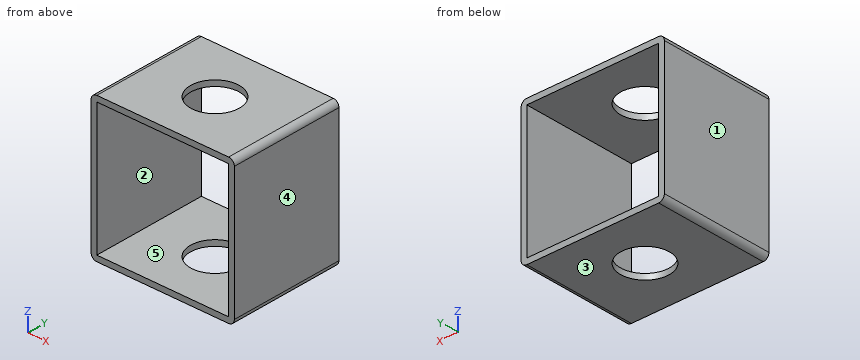
```python
from build123d import *

# Parameters (mm, degrees)
SKETCH1_W               = 46
SKETCH1_H               = 46
EXTRUDE_THIN1_DEPTH     = 20
CUT_EXTRUDE1_DEPTH      = 58.697486947
CUT_EXTRUDE1_DEPTH_BACK = 58.697486947
SKETCH2_R               = 8.5


with BuildPart() as part:
    # Sketch1 → Extrude-Thin1 (new, symmetric)
    with BuildSketch(Plane(origin=(0, 0, 0), x_dir=(1, 0, 0), z_dir=(0, 1, 0))):
        with BuildLine():
            Line((-23, 25), (23, 25))
            ThreePointArc((23, 25), (24.414213562, 24.414213562), (25, 23))
            Line((25, 23), (25, -23))
            ThreePointArc((25, -23), (24.414213562, -24.414213562), (23, -25))
            Line((23, -25), (-23, -25))
            ThreePointArc((-23, -25), (-24.414213562, -24.414213562), (-25, -23))
            Line((-25, -23), (-25, 23))
            ThreePointArc((-25, 23), (-24.414213562, 24.414213562), (-23, 25))
        make_face()
        Rectangle(SKETCH1_W, SKETCH1_H, mode=Mode.SUBTRACT)
    extrude(amount=EXTRUDE_THIN1_DEPTH, both=True)

    # Sketch2 → Cut-Extrude1 (cut, two sides: drawn at the far end of the back side and taken through both)
    with BuildSketch(Plane(origin=(0, 0, 23), x_dir=(-1, 0, 0), z_dir=(0, 0, -1)).offset(-CUT_EXTRUDE1_DEPTH_BACK)):
        Circle(SKETCH2_R)
    extrude(amount=CUT_EXTRUDE1_DEPTH + CUT_EXTRUDE1_DEPTH_BACK, mode=Mode.SUBTRACT)


solid = part.part
```
Here's how the part is built. I have some questions about the finished solid (model axes, mm). Face numbers are marked on the shaded views. A direction names the side the tool comes from. Coordinates: 2 decimals unless noted, no trailing zeros. Loops run counter-clockwise (first coordinate to the right, second up) from the corner with the lowest first, then second, coordinate; pieces in that order, holes last. Notation, with made-up numbers: (34.5, 44) - (87.5, 44) arc R22 ccw to (87.5, 79) - close; hole circle Ø8 at (22.5, -5.5). An arc over 180 degrees is marked (long way). Return JSON: item names as keys, results as strings. Group by question number.
Item 1: If we section it at D-D on x = -21: Write out the boundary of the cut face in (y, z).
Item 2: Will this pin go through, and if not, where does the flat tip stop? P1, Ø19.5, axis at x = 0, y = 0, coming from the -Z side.
Item 3: On a 3-axis mill with a long thin cutter (end or side, diameter ignored), from which of +Z, -Z, +X, -X, +Y, -Y can I reach the whole of each face in a straight line? I mean the marked faces 1 and 2. Say none if no direction works.
Item 4: I need wall thicknesses on line 1 (Z direction, x = -18, y = 13.5); line 2 (Y direction, x = 0, z = -23.65). Which ranges of each line are inside material? Lowest first, please. Write a range as from..to.
Item 5: We'd pull the mould along X, two halves only. Please class the marked faces 3, 4 and 5: +X half, -X half, draft (parallel to the pull), parting line (faces both ways), or undercut.
Item 6: If we section it at A-A on x = 0: Write out the boundary of the cut face in (y, z).
Item 7: If we section it at C-C on z = 6: Write out the boundary of the cut face in (x, y).
Item 8: If we section it at B-B on y = 4: Write out the boundary of the cut face in (x, z), and give its area (3 significant figures).
Calculated:
{
 "1": {"outline": "(-20, -25) - (20, -25) - (20, -23) - (-20, -23) - close; (-20, 23) - (20, 23) - (20, 25) - (-20, 25) - close"},
 "2": {"P1": "stops at z = -25"},
 "3": {"face 1": "+Z, -Z, -X, +Y, -Y", "face 2": "+Y, -Y"},
 "4": {"line 1": "z = -25..-23, 23..25", "line 2": "y = -20..-8.5, 8.5..20"},
 "5": {"face 3": "draft", "face 4": "+X half", "face 5": "undercut"},
 "6": {"outline": "(-20, -25) - (-8.5, -25) - (-8.5, -23) - (-20, -23) - close; (-20, 23) - (-8.5, 23) - (-8.5, 25) - (-20, 25) - close; (8.5, -25) - (20, -25) - (20, -23) - (8.5, -23) - close; (8.5, 23) - (20, 23) - (20, 25) - (8.5, 25) - close"},
 "7": {"outline": "(-25, -20) - (-23, -20) - (-23, 20) - (-25, 20) - close; (23, -20) - (25, -20) - (25, 20) - (23, 20) - close"},
 "8": {"outline": "(-25, -23) arc R2 ccw to (-23, -25) - (-7.5, -25) - (-7.5, -23) - (-23, -23) - (-23, 23) - (-7.5, 23) - (-7.5, 25) - (-23, 25) arc R2 ccw to (-25, 23) - close; (7.5, -25) - (23, -25) arc R2 ccw to (25, -23) - (25, 23) arc R2 ccw to (23, 25) - (7.5, 25) - (7.5, 23) - (23, 23) - (23, -23) - (7.5, -23) - close", "area": "321 mm^2"}
}
